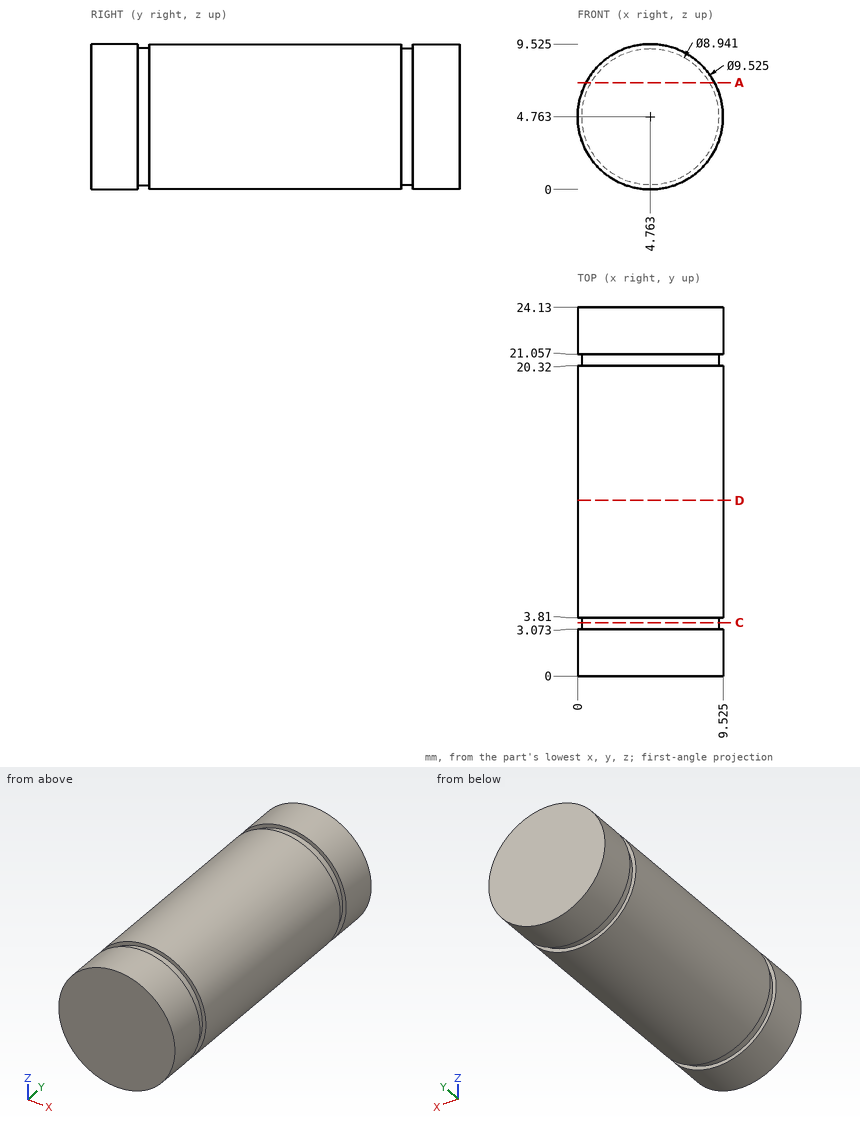
Part print with two shaded views. Sizes in mm from the minimum x, y, z corner. Coordinates: 2 decimals unless noted, no trailing zeros. Order: outer loops, then holes, each group sorted by start corner. A loop starts at its lowest first (then second) coordinate and runs counter-clockwise, first axis right, second up. Notation, with made-up numbers: (69.25, 84.25) - (98.25, 84.25) arc R19 ccw to (98.25, 93.25) - close; hole circle Ø8 at (42, -39.75). An arc over 180 degrees is marked (long way). Answer in a Markdown table with one row per item.
1. Slice it at C-C, the plane y = 3.5. List the corners of the cut face in (x, z), then the cut area to 3 significant figures.
Answer:
| item | result |
|---|---|
| outline | circle Ø8.94 at (4.76, 4.76) |
| area | 62.8 mm² |
2. Flat gauge pins, fed straight in: P1, Ø3, axis at y = 15.5, z = 7, coming from the -X side; P2, Ø1.5, axis at x = 7.5, y = 20.5, coming from the -Z side (1 decimal); P3, Ø4, axis at y = 5.5, z = 2.5, coming from the +X side. Where does each tip first touch, or does it go through?
Answer:
| item | result |
|---|---|
| P1 | x = 0.06 |
| P2 | z = 0.4 |
| P3 | x = 9.52 |
3. Slice it at D-D, the plane y = 11.5. List the corners of the cut face in (x, z) (1 decimal).
Answer:
| item | result |
|---|---|
| outline | circle Ø9.5 at (4.8, 4.8) |
4. Slice it at A-A, the plane z = 7. List the corners of the cut face in (x, y).
Answer:
| item | result |
|---|---|
| outline | (0.56, 0) - (8.97, 0) - (8.97, 3.07) - (8.63, 3.07) - (8.63, 3.81) - (8.97, 3.81) - (8.97, 20.32) - (8.63, 20.32) - (8.63, 21.06) - (8.97, 21.06) - (8.97, 24.13) - (0.56, 24.13) - (0.56, 21.06) - (0.89, 21.06) - (0.89, 20.32) - (0.56, 20.32) - (0.56, 3.81) - (0.89, 3.81) - (0.89, 3.07) - (0.56, 3.07) - close |
5. Drill centre lines: L1, parallel to Y at x = 1, z = 2; L2, parallel to X at y = 5, z = 5 (1 decimal); L3, parallel to X at y = 14.25, z = 9 (1 decimal). Where is each one in solid material? Low to high. Write a range as from..to.
Answer:
| item | result |
|---|---|
| L1 | 0..3.07, 3.81..20.32, 21.06..24.13 |
| L2 | 0..9.5 |
| L3 | 2.6..6.9 |
